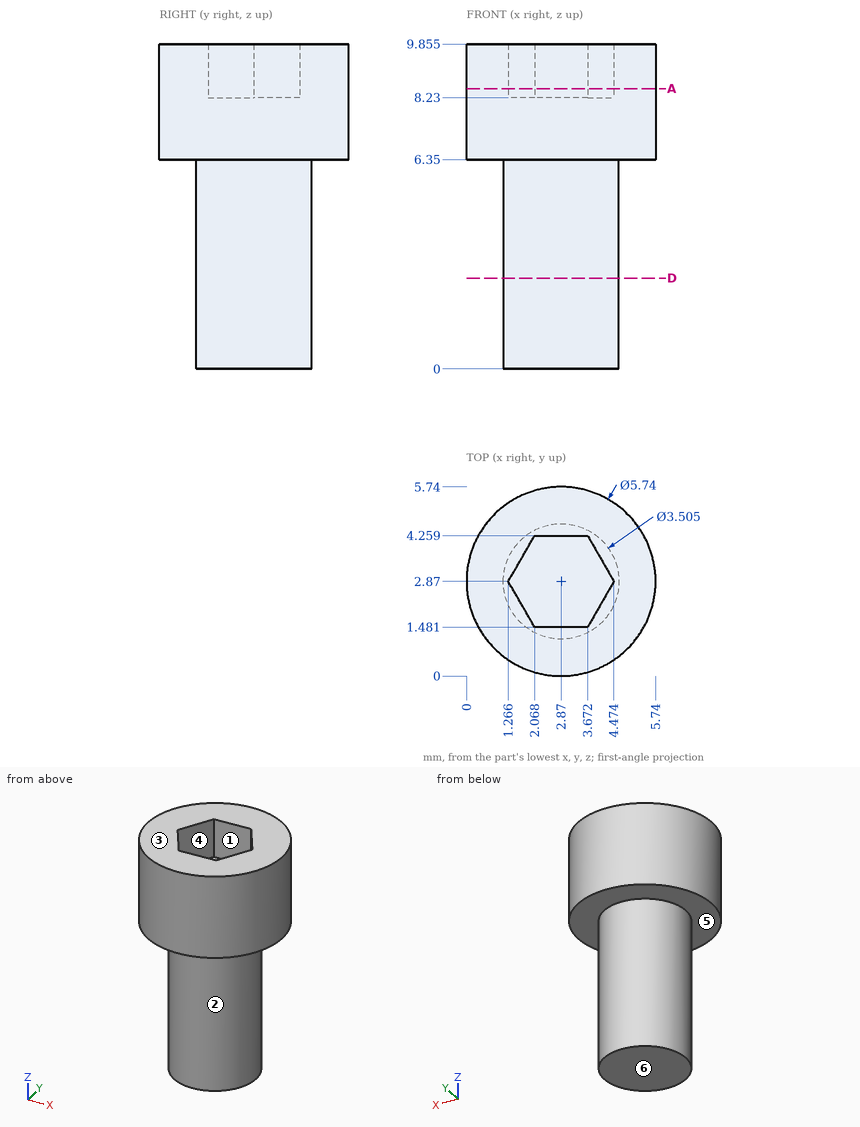
Geometry check sheet. Reference: drawing and pictorial views, mm from the part's lowest x, y, z. A direction names the side the tool comes from. Give positions to 0.01 mm unless a question says otherwise; leave off trailing zeros. Write each loop counter-clockwise with the first axis right and the second up, starting at its lowest first coordinate (ties: lowest second). Pieces come first, ordered by that corner, then holes. Notation, with made-up numbers: (31, -22.5) -> (50, -22.5) arc R19 cw to (50, 9.5) -> close; hole circle Ø1 at (-30.75, -10). An arc over 180 degrees is marked (long way). One line per item, written item: value. Start each with the question number.
Item 1: Tool access check on the marked faces 5 and 6. Record the directions out of +Z, -Z, +X, -X, +Y, -Y that give a thin tool (end or side, any length) a straight path to the whole face; none if there is none.
Item 2: Gauge pin test, flat ends, axial feed: pin 1 (3 mm diameter, centred on y = 2.5, z = 1, fed in from -X); pin 2 (1.5 mm diameter, centred on x = 3.5, z = 1.5, fed in from +Y). Record the tip position at first contact, or that the pin passes through.
Item 3: Section check D-D on z = 2.75. Record the cut outline in (x, y) (1 decimal).
Item 4: Draft check along Y on the marked faces 1, 2, 3 and 4. Enter one of: +Y half, -Y half, draft (parallel to the pull), parting line (faces both ways), or undercut.
Item 5: Section check A-A on z = 8.5. Record the cut outline in (x, y) (1 decimal).
Item 6: Material ranges on probe 1 along Y at (x, z) = (2.85, 8.75); probe 2 along Z at (x, y) = (1.95, 2.6); probe 3 along X at (y, z) = (2.8, 6), recorded low to high. Write a range as from..to.
Results list:
1. face 5: -Z
1. face 6: -Z, +X, -X, +Y, -Y
2. pin 1: x = 1.12
2. pin 2: y = 4.62
3. outline: circle Ø3.5 at (2.9, 2.9)
4. face 1: undercut
4. face 2: parting line
4. face 3: draft
4. face 4: undercut
5. outline: circle Ø5.7 at (2.9, 2.9); hole (1.3, 2.9) -> (2.1, 1.5) -> (3.7, 1.5) -> (4.5, 2.9) -> (3.7, 4.3) -> (2.1, 4.3) -> close
6. probe 1: 0..1.48, 4.26..5.74
6. probe 2: 0..8.23
6. probe 3: 1.12..4.62
